```python
from build123d import *

# Parameters (mm, degrees)
F1_DEPTH = 304.8
F2_START = 50.8
F0_W     = 63.5
F0_H     = 12.7
F2_DEPTH = 254


with BuildPart() as f1:
    # F0 (on Top) → F1 (new body)
    with BuildSketch(Plane.XY):
        Polygon((0, 127), (0, 0), (25.4, 0), (25.4, 12.7), (25.4, 127), align=None)
    extrude(amount=F1_DEPTH)

    # F0 (on Top) → F2 (join)
    with BuildSketch(Plane.XY.offset(F2_START)):
        with Locations((57.15, 6.35)):
            Rectangle(F0_W, F0_H)
    extrude(amount=F2_DEPTH)


solid = f1.part
```
Input: part model. Units: mm. Frame: model coordinates. A direction names the side the tool comes from. Give positions to 0.01 mm unless a question says otherwise; leave off trailing zeros. Write each loop counter-clockwise with the first axis right and the second up, starting at its lowest first coordinate (ties: lowest second). Pieces come first, ordered by that corner, then holes. Notation, with made-up numbers: (16, 42.25) - (60, 42.25) arc R11 ccw to (60, 51.25) - close; hole circle Ø11 at (80.5, 84). An arc over 180 degrees is marked (long way). Write item = value, one per line. Start each with the question number.
1. First-contact query: pin 1 Ø4 at (y, z) = (97, 60.5) entering from +X; pin 2 Ø4 at (x, y) = (55.5, 5) entering from -Z; pin 3 Ø5 at (x, z) = (59.5, 254.5) entering from +Y. Flat tips, straight axial feed; report the tip coordinate or a pass-through.
2. Section query C-C, the plane y = 87.5. Output: boundary loops of the cut face in (x, z), then the cut area to 3 significant figures.
3. Access query for faces 1 (the flat face through (57, 6, 50.8)), 2 (the flat face through (57, 12.7, 176)), 3 (the flat face through (44, 0, 184)). Directions: +Z, -Z, +X, -X, +Y, -Y. A direction counts if a zero-diameter tool reaches every point of the face in a straight line with its end or side. Return the directions, or none.
4. Section query A-A, the plane z = 122.5. Output: boundary loops of the cut face in (x, y), then the cut area to 3 significant figures.
5. Ray query, L1, parallel to X at y = 91.5, z = 214.5; L2, parallel to Y at x = 31.5, z = 145. Return the intervals inside material, ascending.
6. Section query B-B, the plane x = 31. Output: boundary loops of the cut face in (y, z).
Check sheet entries:
q1.pin_1 = 25.4
q1.pin_2 = 50.8
q1.pin_3 = 12.7
q2.outline = (0, 0) - (25.4, 0) - (25.4, 304.8) - (0, 304.8) - close
q2.area = 7,740 mm2
q3.face_1 = -Z, +X, +Y, -Y
q3.face_2 = +Z, -Z, +X, +Y
q3.face_3 = +Z, -Z, +X, -X, -Y
q4.outline = (0, 0) - (88.9, 0) - (88.9, 12.7) - (25.4, 12.7) - (25.4, 127) - (0, 127) - close
q4.area = 4,030 mm2
q5.L1 = 0 to 25.4
q5.L2 = 0 to 12.7
q6.outline = (0, 50.8) - (12.7, 50.8) - (12.7, 304.8) - (0, 304.8) - close
